```python
from build123d import *

# Parameters (mm, degrees)
SKETCH1_R                = 1.175
BOSS_EXTRUDE1_DEPTH      = 6.4
SKETCH2_W                = 1
SKETCH2_H                = 3.6
BOSS_EXTRUDE2_DEPTH      = 1
SKETCH3_W                = 0.3
SKETCH3_H                = 3.2
BOSS_EXTRUDE3_DEPTH      = 3.9
SKETCH4_R                = 0.8
CUT_EXTRUDE1_DEPTH       = 23.144976857
BOSS_EXTRUDE4_DEPTH      = 0.25
BOSS_EXTRUDE4_DEPTH_BACK = 6.65
SKETCH5_R                = 1.175
FILLET1_R                = 0.5
FILLET2_R                = 0.25
FILLET3_R                = 0.25


with BuildPart() as part:
    # Sketch1 → Boss-Extrude1 (new body)
    with BuildSketch(Plane.XY):
        Polygon((0, 0), (-3.95, 0), (-3.95, -0.4), (-6.45, -0.4), (-6.45, 0), (-13.45, 0), (-13.45, -0.4), (-15.95, -0.4), (-15.95, 0), (-19.8, 0), (-19.8, 10.2), (-10.1, 10.2), (-9.4, 9.5), (0, 9.5), align=None)
        with Locations((-14.7, 2.5)):
            Circle(SKETCH1_R, mode=Mode.SUBTRACT)
        with Locations((-5.2, 2.5)):
            Circle(SKETCH1_R, mode=Mode.SUBTRACT)
    extrude(amount=BOSS_EXTRUDE1_DEPTH)

    # Sketch2 → Boss-Extrude2 (add)
    with BuildSketch(Plane(origin=(0, 10.2, 0), x_dir=(1, 0, 0), z_dir=(0, 1, 0))):
        with Locations((-11.1, -3.2)):
            Rectangle(SKETCH2_W, SKETCH2_H)
    extrude(amount=BOSS_EXTRUDE2_DEPTH)

    # Sketch3 → Boss-Extrude3 (add)
    with BuildSketch(Plane.XZ):
        with Locations((-18.05, 3.2)):
            Rectangle(SKETCH3_W, SKETCH3_H)
        with Locations((-9.25, 3.2)):
            Rectangle(SKETCH3_W, SKETCH3_H)
        with Locations((-1.95, 3.2)):
            Rectangle(SKETCH3_W, SKETCH3_H)
    extrude(amount=BOSS_EXTRUDE3_DEPTH)

    # Sketch4 → Cut-Extrude1 (cut, through all)
    with BuildSketch(Plane(origin=(-1.8, 0, 0), x_dir=(0, 0, -1), z_dir=(1, 0, 0))):
        with Locations(Location((-3.2, -2.3, 0), (0, 0, 90))):
            Circle(SKETCH4_R)
    extrude(amount=-CUT_EXTRUDE1_DEPTH, mode=Mode.SUBTRACT)

    # Sketch5 → Boss-Extrude4 (add, two sides: drawn at the far end of the back side and taken through both)
    # profile 1 of 2: a face of its own
    with BuildSketch(Plane.XY.offset(6.4).offset(-BOSS_EXTRUDE4_DEPTH_BACK)):
        with BuildLine():
            Line((-16.175, 2.5), (-16.175, 0))
            Line((-16.175, 0), (-15.95, 0))
            Line((-15.95, 0), (-15.95, -0.4))
            Line((-15.95, -0.4), (-13.45, -0.4))
            Line((-13.45, -0.4), (-13.45, 0))
            Line((-13.45, 0), (-13.225, 0))
            Line((-13.225, 0), (-13.225, 2.5))
            ThreePointArc((-13.225, 2.5), (-14.7, 3.975), (-16.175, 2.5))
        make_face()
        with Locations(Location((-14.7, 2.5, 0), (0, 0, 180))):
            Circle(SKETCH5_R, mode=Mode.SUBTRACT)
    # profile 2 of 2: a face of its own
    with BuildSketch(Plane.XY.offset(6.4).offset(-BOSS_EXTRUDE4_DEPTH_BACK)):
        with BuildLine():
            Line((-6.675, 2.5), (-6.675, 0))
            Line((-6.675, 0), (-6.45, 0))
            Line((-6.45, 0), (-6.45, -0.4))
            Line((-6.45, -0.4), (-3.95, -0.4))
            Line((-3.95, -0.4), (-3.95, 0))
            Line((-3.95, 0), (-3.725, 0))
            Line((-3.725, 0), (-3.725, 2.5))
            ThreePointArc((-3.725, 2.5), (-5.2, 3.975), (-6.675, 2.5))
        make_face()
        with Locations(Location((-5.2, 2.5, 0), (0, 0, 180))):
            Circle(SKETCH5_R, mode=Mode.SUBTRACT)
    extrude(amount=BOSS_EXTRUDE4_DEPTH + BOSS_EXTRUDE4_DEPTH_BACK)

    # Fillet1
    # the kernel refuses this fillet: 0.5 mm, written as the material it takes off along each edge
    with BuildSketch(Plane(origin=(-19.8, 10.2, -1.25), x_dir=(0, -1, 0), z_dir=(0, 0, 1)), Plane(origin=(0, 9.5, -1.25), x_dir=(-1, 0, 0), z_dir=(0, 0, 1))) as fillet1_piece_1:
        with BuildLine():
            CenterArc((FILLET1_R, FILLET1_R), FILLET1_R, 180, 90)
            Line((0, FILLET1_R), (-FILLET1_R * 0.02, FILLET1_R))
            Line((-FILLET1_R * 0.02, FILLET1_R), (-FILLET1_R * 0.02, -FILLET1_R * 0.02))
            Line((-FILLET1_R * 0.02, -FILLET1_R * 0.02), (FILLET1_R, -FILLET1_R * 0.02))
            Line((FILLET1_R, -FILLET1_R * 0.02), (FILLET1_R, 0))
        make_face()
    extrude(amount=8.9, mode=Mode.SUBTRACT)
    with BuildSketch(Plane(origin=(-3.95, -0.4, 7.874744871), x_dir=(-1, 0, 0), z_dir=(0, 0, -1))) as fillet1_piece_2:
        with BuildLine():
            CenterArc((0.489897949, 0.5), FILLET1_R, 191.536959033, 78.463040967)
            Line((0, 0.4), (-0.009797959, 0.398))
            ThreePointArc((-0.009797959, 0.398), (-0.01, 0.2), (-0.01, 0))
            Line((-0.01, 0), (0, -0.01))
            Line((0, -0.01), (0.489897949, -0.01))
            Line((0.489897949, -0.01), (0.489897949, 0))
        make_face()
    extrude(amount=9.349489743, mode=Mode.SUBTRACT)
    with BuildSketch(Plane(origin=(-6.45, -0.4, 0), x_dir=(1, 0, 0), z_dir=(0, 0, 1))) as fillet1_piece_3:
        with BuildLine():
            CenterArc((0.489897949, 0.5), FILLET1_R, 191.536959033, 78.463040967)
            Line((0, 0.4), (-0.009797959, 0.398))
            ThreePointArc((-0.009797959, 0.398), (-0.01, 0.2), (-0.01, 0))
            Line((-0.01, 0), (0, -0.01))
            Line((0, -0.01), (0.489897949, -0.01))
            Line((0.489897949, -0.01), (0.489897949, 0))
        make_face()
    extrude(amount=6.4, mode=Mode.SUBTRACT)
    with BuildSketch(Plane(origin=(-13.45, -0.4, -1.474744871), x_dir=(-1, 0, 0), z_dir=(0, 0, 1))) as fillet1_piece_4:
        with BuildLine():
            CenterArc((0.489897949, -0.5), FILLET1_R, 90, 78.463040967)
            Line((0, -0.4), (-0.009797959, -0.398))
            ThreePointArc((-0.009797959, -0.398), (-0.01, -0.2), (-0.01, 0))
            Line((-0.01, 0), (0, 0.01))
            Line((0, 0.01), (0.489897949, 0.01))
            Line((0.489897949, 0.01), (0.489897949, 0))
        make_face()
    extrude(amount=9.349489743, mode=Mode.SUBTRACT)
    with BuildSketch(Plane(origin=(-15.95, -0.4, -1.474744871), x_dir=(0, 1, 0), z_dir=(0, 0, 1))) as fillet1_piece_5:
        with BuildLine():
            CenterArc((0.5, -0.489897949), FILLET1_R, 101.536959033, 78.463040967)
            Line((0, -0.489897949), (-0.01, -0.489897949))
            Line((-0.01, -0.489897949), (-0.01, 0))
            Line((-0.01, 0), (0, 0.01))
            ThreePointArc((0, 0.01), (0.2, 0.01), (0.398, 0.009797959))
            Line((0.398, 0.009797959), (0.4, 0))
        make_face()
    extrude(amount=9.349489743, mode=Mode.SUBTRACT)
    with BuildSketch(Plane(origin=(-6.45, -0.4, -1.474744871), x_dir=(1, 0, 0), z_dir=(0, 0, 1))) as fillet1_piece_6:
        with BuildLine():
            CenterArc((0.489897949, 0.5), FILLET1_R, 191.536959033, 78.463040967)
            Line((0, 0.4), (-0.009797959, 0.398))
            ThreePointArc((-0.009797959, 0.398), (-0.01, 0.2), (-0.01, 0))
            Line((-0.01, 0), (0, -0.01))
            Line((0, -0.01), (0.489897949, -0.01))
            Line((0.489897949, -0.01), (0.489897949, 0))
        make_face()
    extrude(amount=1.474744871, mode=Mode.SUBTRACT)
    with BuildSketch(Plane(origin=(-6.45, -0.4, 6.4), x_dir=(1.578737141016463e-12, 1.0, 0), z_dir=(0, 0, 1))) as fillet1_piece_7:
        with BuildLine():
            CenterArc((0.5, -0.489897949), FILLET1_R, 101.536959033, 78.463040967)
            Line((0, -0.489897949), (-0.01, -0.489897949))
            Line((-0.01, -0.489897949), (-0.01, 0))
            Line((-0.01, 0), (0, 0.01))
            ThreePointArc((0, 0.01), (0.2, 0.01), (0.398, 0.009797959))
            Line((0.398, 0.009797959), (0.4, 0))
        make_face()
    extrude(amount=1.474744871, mode=Mode.SUBTRACT)

    # Fillet2
    fillet2_edges = [part.edges().sort_by_distance(p)[0] for p in [
        (-18.05, -3.9, 1.6),
        (-18.05, -3.9, 4.8),
        (-9.25, -3.9, 1.6),
        (-9.25, -3.9, 4.8),
        (-1.95, -3.9, 1.6),
        (-1.95, -3.9, 4.8),
    ]]
    fillet(fillet2_edges, radius=FILLET2_R)

    # Fillet3
    fillet3_edges = [part.edges().sort_by_distance(p)[0] for p in [
        (-11.6, 11.2, 3.2),
        (-10.6, 11.2, 3.2),
    ]]
    fillet(fillet3_edges, radius=FILLET3_R)


solid = part.part
```
Check sheet for the modelled part. Datum: model origin and axes. Units: mm. A direction names the side the tool comes from. Round coordinates to 2 decimals unless told otherwise and drop trailing zeros. Order: outer loops, then holes, each group sorted by start corner. A loop starts at its lowest first (then second) coordinate and runs counter-clockwise, first axis right, second up. Notation, with made-up numbers: (-33, 7) -> (-20, 7) arc R25 ccw to (-20, 39) -> close; hole circle Ø8 at (67.25, -38). An arc over 180 degrees is marked (long way). One line per item, written item: value. Start each with the question number.
Q1. Mould release check, pull along X, two halves, no side actions. Record for faces 1 (the face through (-1.8, -1, 3)), 2 (the face through (-9.4, -1, 3)), 3 (the face through (-5, 1, 6.65)): pulls with the +X half, pulls with the -X half, needs draft (parallel to the pull), parting line crosses it, or undercut.
Q2. Cross-section at B-B (y = -2.3). Record the boundary of the cut face in (x, z), and give its area (3 significant figures).
Q3. Gauge pin test, flat ends, axial feed: pin 1 Ø1.6 at (y, z) = (-2, 3) entering from +X; pin 2 Ø2.5 at (y, z) = (-2.3, 3.2) entering from -X; pin 3 Ø0.8 at (x, z) = (-5, 1.5) entering from -Y. Record the tip position at first contact, or that the pin passes through.
Q4. Set-up check for faces 4 (the face through (-11, 11, 5)), 5 (the face through (-15, -0.4, 3)), 6 (the face through (-5, 9.5, 3)), 7 (the face through (-18.05, -2.89, 3.74)), 8 (the face through (-11, 11, 1.4)): record each of +Z, -Z, +X, -X, +Y, -Y from which the full face is reachable in a straight line by a thin tool's end or side.
Q5. Cross-section at C-C (z = 5.25). Record the boundary of the cut face in (x, y) (3 decimals).
Q6. Cross-section at A-A (x = -14.7). Record the boundary of the cut face in (y, z) (3 decimals).
Q7. Cross-section at D-D (y = 2). Record the boundary of the cut face in (x, z) (3 decimals).
Q8. Thickness scan on line 1 (X direction, y = 2.5, z = 4.25) (3 decimals); line 2 (Y direction, x = -14.7, z = 3.5) (3 decimals); line 3 (Z direction, x = -18, y = -2.3). Record the ranges inside material, lowest first.
Completed:
1. face 1: pulls with the +X half
1. face 2: undercut
1. face 3: needs draft
2. outline: (-18.2, 1.6) -> (-17.9, 1.6) -> (-17.9, 2.4) -> (-18.2, 2.4) -> close; (-18.2, 4) -> (-17.9, 4) -> (-17.9, 4.8) -> (-18.2, 4.8) -> close; (-9.4, 1.6) -> (-9.1, 1.6) -> (-9.1, 2.4) -> (-9.4, 2.4) -> close; (-9.4, 4) -> (-9.1, 4) -> (-9.1, 4.8) -> (-9.4, 4.8) -> close; (-2.1, 1.6) -> (-1.8, 1.6) -> (-1.8, 2.4) -> (-2.1, 2.4) -> close; (-2.1, 4) -> (-1.8, 4) -> (-1.8, 4.8) -> (-2.1, 4.8) -> close
2. area: 1.44 mm²
3. pin 1: stops at x = -1.8
3. pin 2: stops at x = -18.2
3. pin 3: stops at y = -0.4
4. face 4: +Z, +X, -X, +Y
4. face 5: +Z, -Z, -Y
4. face 6: +Z, -Z, +X, +Y
4. face 7: +X, -X
4. face 8: -Z, +X, -X, +Y
5. outline: (-19.8, 0) -> (-15.95, 0) arc R0.5 ccw to (-15.46, -0.4) -> (-13.94, -0.4) arc R0.5 ccw to (-13.45, 0) -> (-6.45, 0) arc R0.5 ccw to (-5.96, -0.4) -> (-4.44, -0.4) arc R0.5 ccw to (-3.95, 0) -> (0, 0) -> (0, 9) arc R0.5 ccw to (-0.5, 9.5) -> (-9.4, 9.5) -> (-10.1, 10.2) -> (-19.3, 10.2) arc R0.5 ccw to (-19.8, 9.7) -> close; hole circle Ø2.35 at (-14.7, 2.5); hole circle Ø2.35 at (-5.2, 2.5)
6. outline: (-0.4, -0.25) -> (1.325, -0.25) -> (1.325, 6.65) -> (-0.4, 6.65) -> close; (3.675, -0.25) -> (3.975, -0.25) -> (3.975, 0) -> (10.2, 0) -> (10.2, 6.4) -> (3.975, 6.4) -> (3.975, 6.65) -> (3.675, 6.65) -> close
7. outline: (-19.8, 0) -> (-16.175, 0) -> (-16.175, -0.25) -> (-15.763, -0.25) -> (-15.763, 6.65) -> (-16.175, 6.65) -> (-16.175, 6.4) -> (-19.8, 6.4) -> close; (-13.637, -0.25) -> (-13.225, -0.25) -> (-13.225, 0) -> (-6.675, 0) -> (-6.675, -0.25) -> (-6.263, -0.25) -> (-6.263, 6.65) -> (-6.675, 6.65) -> (-6.675, 6.4) -> (-13.225, 6.4) -> (-13.225, 6.65) -> (-13.637, 6.65) -> close; (-4.137, -0.25) -> (-3.725, -0.25) -> (-3.725, 0) -> (0, 0) -> (0, 6.4) -> (-3.725, 6.4) -> (-3.725, 6.65) -> (-4.137, 6.65) -> close
8. line 1: x = -19.8 to -15.875, -13.525 to -6.375, -4.025 to 0
8. line 2: y = -0.4 to 1.325, 3.675 to 10.2
8. line 3: z = 1.6 to 2.4, 4 to 4.8
